Verification items for this drawing (mm, ordinates from the low corner). A direction names the side the tool comes from. Give positions to 0.01 mm unless a question says otherwise; leave off trailing zeros. Loops run counter-clockwise (first coordinate to the right, second up) from the corner with the lowest first, then second, coordinate; pieces in that order, holes last. Notation, with made-up numbers: M 40,70.5 L 78,70.5 A21 ccw 78,95.5 Z; hole C -21,54 d5. An arc over 180 degrees is marked long. Use one line per item in the form item = value.
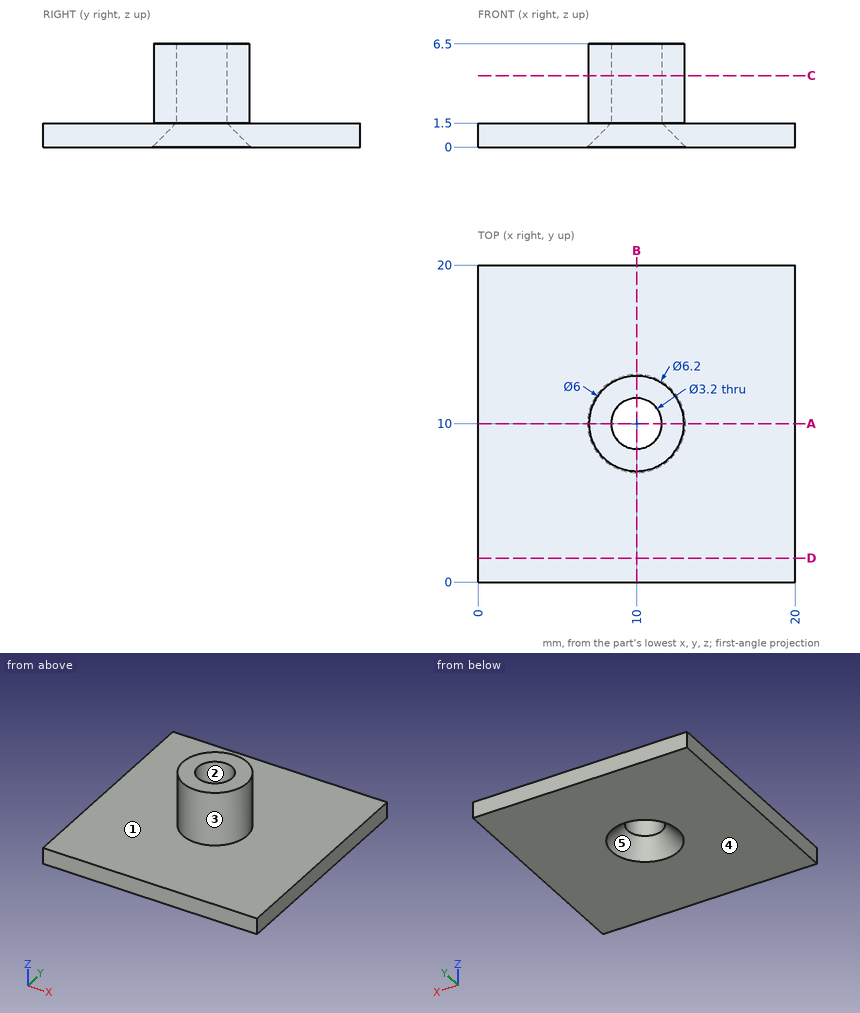
1) Section check D-D (y = 1.5). Record the cut outline in (x, z).
Evaluation:
outline = M 0,0 L 20,0 L 20,1.5 L 0,1.5 Z
2) Release check for a two-part mould opening along X. For the marked faces 3, 4 and 5 record: pulls with the +X half, pulls with the -X half, needs draft (parallel to the pull), parting line crosses it, or undercut.
Evaluation:
face_3 = parting line crosses it
face_4 = needs draft
face_5 = undercut
3) Scan lines: line 1 (Y direction, x = 10, z = 3); line 2 (Z direction, x = 10.5, y = 2.5); line 3 (X direction, y = 10.5, z = 2). Record each from-to range of solid material in increasing order.
Evaluation:
line_1 = 7 to 8.4, 11.6 to 13
line_2 = 0 to 1.5
line_3 = 7.04 to 8.48, 11.52 to 12.96
4) Section check C-C (z = 4.5). Record the cut outline in (x, y).
Evaluation:
outline = C 10,10 d6; hole C 10,10 d3.2
5) Set-up check for the marked faces 1 and 2: record each of +Z, -Z, +X, -X, +Y, -Y from which the full face is reachable in a straight line by a thin tool's end or side.
Evaluation:
face_1 = +Z
face_2 = +Z, -Z
6) Depth check by flat-ended pin: pin 1 Ø2 at (y, z) = (16, 4) entering from -X; pin 2 Ø1 at (x, y) = (7.5, 7.5) entering from +Z; pin 3 Ø3 at (y, z) = (14, 4.5) entering from +X. Enter the tip coordinate at first touch or a pass-through.
Evaluation:
pin_1 = through
pin_2 = 1.5
pin_3 = 11.66
7) Section check A-A (y = 10). Record the cut outline in (x, z), then the cut area to 4 significant figures.
Evaluation:
outline = M 0,0 L 6.9,0 L 8.4,1.5 L 8.4,6.5 L 7,6.5 L 7,1.5 L 0,1.5 Z; M 11.6,1.5 L 13.1,0 L 20,0 L 20,1.5 L 13,1.5 L 13,6.5 L 11.6,6.5 Z
area = 36.95 mm^2
